from build123d import *

# Parameters (mm, degrees)
F0_R     = 30
F1_DEPTH = 13.75
F2_R     = 30
F2_R_2   = 27.75
F3_DEPTH = 18.25
F5_D     = 13.67
F5_DEPTH = 13.75


with BuildPart() as f1:
    # F0 (on Top) → F1 (new body)
    with BuildSketch(Plane.XY):
        Circle(F0_R)
    extrude(amount=F1_DEPTH)

    # F2 (on face) → F3 (join)
    with BuildSketch(Plane.XY.offset(13.75)):
        Circle(F2_R)
        Circle(F2_R_2, mode=Mode.SUBTRACT)
    extrude(amount=F3_DEPTH)

    # F5
    with Locations(Plane(origin=(0, 0, 0), x_dir=(1, 0, 0), z_dir=(0, 0, -1))):
        with Locations((0, 0)):
            Hole(F5_D / 2, depth=F5_DEPTH)


solid = f1.part
Input: part model. Units: mm. Frame: model coordinates. A direction names the side the tool comes from. Round coordinates to 2 decimals unless told otherwise and drop trailing zeros. Order: outer loops, then holes, each group sorted by start corner. A loop starts at its lowest first (then second) coordinate and runs counter-clockwise, first axis right, second up. Notation, with made-up numbers: (-10, -18.5) - (18, -18.5) arc R33 cw to (18, 15.5) - close; hole circle Ø7 at (25, -38.75). An arc over 180 degrees is marked (long way). Use a Markdown table: item, result.
1. Section A-A on x = 0. Return the cut outline in (y, z) (3 decimals), then the cut area to 3 significant figures.
Evaluation:
| item | result |
|---|---|
| outline | (-30, 0) - (-6.835, 0) - (-6.835, 13.75) - (-27.75, 13.75) - (-27.75, 32) - (-30, 32) - close; (6.835, 0) - (30, 0) - (30, 32) - (27.75, 32) - (27.75, 13.75) - (6.835, 13.75) - close |
| area | 719 mm^2 |
2. Access query for faces 4 (the face through (9, -27, 32)), 5 (the face through (26.469, 8.335, 22.747)). Directions: +Z, -Z, +X, -X, +Y, -Y. A direction counts if a zero-diameter tool reaches every point of the face in a straight line with its end or side. Return the directions, or none.
Evaluation:
| item | result |
|---|---|
| face 4 | +Z, +X, -X, +Y, -Y |
| face 5 | +Z |
3. Mould query, pull axis X, two halves, no side actions, for faces 1 (the face through (0, 7, 0)), 2 (the face through (-29.97, 1.32, 15.78)), 3 (the face through (1.482, 6.672, 6.971)). Classes: +X half, -X half, draft (parallel to the pull), parting line (faces both ways), or undercut.
Evaluation:
| item | result |
|---|---|
| face 1 | draft |
| face 2 | parting line |
| face 3 | undercut |
4. First-contact query: pin 1 (16.5 mm diameter, centred on x = -12, y = 8, fed in from +Z); pin 2 (1 mm diameter, centred on y = 3, z = 6, fed in from -X); pin 3 (10 mm diameter, centred on y = 9, z = 8, fed in from +X). Flat tips, straight axial feed; report the tip coordinate or a pass-through.
Evaluation:
| item | result |
|---|---|
| pin 1 | z = 13.75 |
| pin 2 | x = -29.9 |
| pin 3 | x = 29.73 |
5. Section C-C on z = 4. Return the cut outline in (x, y) (3 decimals), then the cut area to 3 significant figures.
Evaluation:
| item | result |
|---|---|
| outline | circle Ø60 at (0, 0); hole circle Ø13.67 at (0, 0) |
| area | 2,680 mm^2 |
6. Material intervals for probe 1 along Y at (x, z) = (0, 23.5); probe 2 along Y at (x, z) = (0, 10.25) (3 decimals); probe 3 along X at (y, z) = (-4.5, 12), sorted ascending.
Evaluation:
| item | result |
|---|---|
| probe 1 | -30 to -27.75, 27.75 to 30 |
| probe 2 | -30 to -6.835, 6.835 to 30 |
| probe 3 | -29.66 to -5.14, 5.14 to 29.66 |
7. Section D-D on y = -14.5. Return the cut outline in (x, z).
Evaluation:
| item | result |
|---|---|
| outline | (-26.26, 0) - (26.26, 0) - (26.26, 32) - (23.66, 32) - (23.66, 13.75) - (-23.66, 13.75) - (-23.66, 32) - (-26.26, 32) - close |
